Read the model definition and answer for the solid it produces. Units are mm, in the model's axes. A direction names the side the tool comes from. Coordinates: 2 decimals unless noted, no trailing zeros. Loops run counter-clockwise (first coordinate to the right, second up) from the corner with the lowest first, then second, coordinate; pieces in that order, holes last. Notation, with made-up numbers: (-27, -1) -> (-4, -1) arc R18 ccw to (-4, 29) -> close; hole circle Ø8 at (34.25, -27.75). An arc over 180 degrees is marked (long way). Answer as CSV lines item,"result".
```python
from build123d import *

# Parameters (mm, degrees)
SKETCH_R     = 3
PAD_DEPTH    = 12
SKETCH001_R  = 6
PAD001_DEPTH = 80
FILLET_R     = 2


with BuildPart() as part:
    # Sketch → Pad (new body)
    with BuildSketch(Plane.XY):
        Circle(SKETCH_R)
        Polygon((2.2, 0), (1.1, 1.905256), (-1.1, 1.905256), (-2.2, 0), (-1.1, -1.905256), (1.1, -1.905256), align=None, mode=Mode.SUBTRACT)
    extrude(amount=PAD_DEPTH)

    # Sketch001 (on Face9 of Pad) → Pad001 (join)
    with BuildSketch(Plane.XY.offset(12)):
        Circle(SKETCH001_R)
    extrude(amount=PAD001_DEPTH)

    # Fillet
    fillet_edges = [part.edges().sort_by_distance(p)[0] for p in [
        (-6, 0, 12),
    ]]
    fillet(fillet_edges, radius=FILLET_R)


solid = part.part
```
Q1. Given pin 1 Ø1 at (y, z) = (1, 39.5) entering from +X; pin 2 Ø1.8 at (x, z) = (0.5, 5.5) entering from -Y; pin 3 Ø4 at (x, y) = (0, 1) entering from -Z; pin 4 Ø5 at (x, z) = (3.5, 31) entering from +Y, each flat-ended and moving along its own axis, determine where each tip first touches the part or whether it passes through.
Results:
pin 1,"stops at x = 5.98"
pin 2,"stops at y = -3"
pin 3,"stops at z = 0"
pin 4,"stops at y = 5.92"
Q2. For a pull along Y with two mould halves and no side action, classify faces 1 (the face through (1, 3, 12)), 2 (the face through (-1.64, 0.97, 5.92)), 3 (the face through (-6, 0, 52)) as pulls with the +Y half, pulls with the -Y half, needs draft (parallel to the pull), parting line crosses it, or undercut.
Results:
face 1,"needs draft"
face 2,"undercut"
face 3,"parting line crosses it"
Q3. Find the intervals of material crossed by probe 1 along Z at (x, y) = (1, 0.25); probe 2 along X at (y, z) = (0.25, 27); probe 3 along Y at (x, z) = (-4.25, 23.5), in increasing order. Write a range as [from, to].
Results:
probe 1,"z = [12, 92]"
probe 2,"x = [-5.99, 5.99]"
probe 3,"y = [-4.24, 4.24]"
Q4. A cutting plane is placed at A-A, the plane x = 0. Write down the section's boundary in (y, z).
Results:
outline,"(-6, 14) arc R2 ccw to (-4, 12) -> (-3, 12) -> (-3, 0) -> (-1.91, 0) -> (-1.91, 12) -> (1.91, 12) -> (1.91, 0) -> (3, 0) -> (3, 12) -> (4, 12) arc R2 ccw to (6, 14) -> (6, 92) -> (-6, 92) -> close"
Q5. For faces 4 (the face through (2, -1, 0)), 5 (the face through (0, 1.905, 6)), determine the directions among +Z, -Z, +X, -X, +Y, -Y from which every point of the face is accessible in a straight line to the end or side of a thin tool.
Results:
face 4,"-Z, +X, -X, +Y, -Y"
face 5,"-Z"
Q6. A cutting plane is placed at B-B, the plane z = 83. Write down the section's boundary in (x, y).
Results:
outline,"circle Ø12 at (0, 0)"
